from build123d import *

# Parameters (mm, degrees)
SKETCH1_W           = 10
SKETCH1_H           = 10
SKETCH1_W_2         = 8
SKETCH1_H_2         = 8
BOSS_EXTRUDE1_DEPTH = 200
FILLET2_R           = 1
SKETCH2_R           = 3.75
SKETCH2_R_2         = 2.25
CUT_EXTRUDE1_DEPTH  = 201.31225624


with BuildPart() as part:
    # Sketch1 → Boss-Extrude1 (new body)
    with BuildSketch(Plane(origin=(0, 0, 0), x_dir=(1, 0, 0), z_dir=(0, 1, 0))):
        Rectangle(SKETCH1_W, SKETCH1_H)
        Rectangle(SKETCH1_W_2, SKETCH1_H_2, mode=Mode.SUBTRACT)
    extrude(amount=BOSS_EXTRUDE1_DEPTH)

    # Fillet2
    fillet2_edges = [part.edges().sort_by_distance(p)[0] for p in [
        (4, 0, 0),
        (0, 0, -4),
        (-4, 0, 0),
        (0, 0, 4),
        (4, 200, 0),
        (0, 200, -4),
        (-4, 200, 0),
        (0, 200, 4),
    ]]
    fillet(fillet2_edges, radius=FILLET2_R - 0.0001)  # a hair under: the kernel refuses the full size

    # Sketch2 → Cut-Extrude1 (cut, through all)
    with BuildSketch(Plane.XY.offset(5)):
        with Locations((0, 10)):
            Circle(SKETCH2_R)
        with Locations((0, 190)):
            Circle(SKETCH2_R_2)
    extrude(amount=-CUT_EXTRUDE1_DEPTH, mode=Mode.SUBTRACT)


solid = part.part
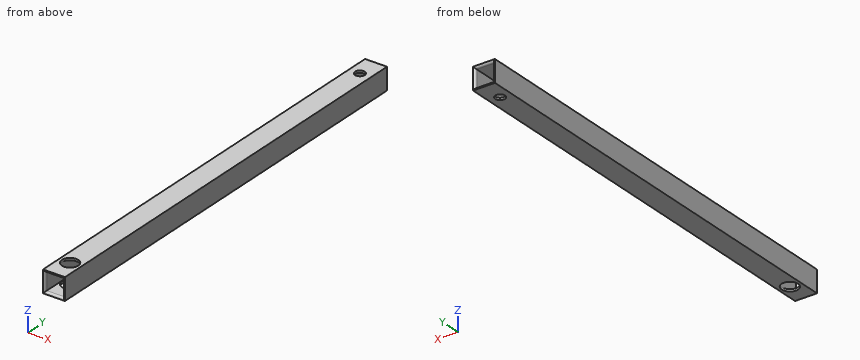
Build history of the part. All positions in model axes, mm. Round coordinates to 2 decimals unless told otherwise and drop trailing zeros. Write each loop counter-clockwise with the first axis right and the second up, starting at its lowest first coordinate (ties: lowest second). Pieces come first, ordered by that corner, then holes. Notation, with made-up numbers: (22, 73.5) -> (65, 73.5) arc R25 cw to (65, 95.5) -> close; hole circle Ø6 at (21, 52.5). An arc over 180 degrees is marked (long way). Use one line per item in the form item = value.
Q1. Drill centre lines: L1, parallel to Z at x = 3, y = 60; L2, parallel to X at y = 190, z = -4.45. Where is each one in solid material? Low to high.
Conclusion:
L1 = -5 to -4, 4 to 5
L2 = -5 to -2.25, 2.25 to 5
Q2. Drop a flat-ended pin along its axis: P1, Ø6, axis at x = 0, y = 190, coming from the -Z side. Give the stop position or say it passes through.
Conclusion:
P1 = -5
Q3. Band-saw the part on B-B, the plane x = 0. State how many separate pieces and enclosed holes the cut face has, then the cut area to 3 significant figures.
Conclusion:
separate_pieces = 6
enclosed_holes = 0
area = 375 mm²
Q4. Band-saw the part on A-A, the plane y = 10. Write the cut outline in (x, z).
Conclusion:
outline = (-5, -5) -> (-3.75, -5) -> (-3.75, -4) -> (-4, -4) -> (-4, 4) -> (-3.75, 4) -> (-3.75, 5) -> (-5, 5) -> close; (3.75, -5) -> (5, -5) -> (5, 5) -> (3.75, 5) -> (3.75, 4) -> (4, 4) -> (4, -4) -> (3.75, -4) -> close
Q5. Band-saw the part on D-D, the plane y = 174.5. Write the cut outline in (x, z).
Conclusion:
outline = (-5, -5) -> (5, -5) -> (5, 5) -> (-5, 5) -> close; hole (-4, -4) -> (4, -4) -> (4, 4) -> (-4, 4) -> close
